```python
from build123d import *

# Parameters (mm, degrees)
SKETCH_R          = 20.32
SKETCH_R_2        = 2.225
PAD_DEPTH         = 36.83
FILLET_R          = 0.5
SKETCH001_R       = 1.05
PAD001_DEPTH      = 18.415
PAD001_DEPTH_BACK = 3.5


with BuildPart() as fillet_body:
    # Sketch → Pad (new body)
    with BuildSketch(Plane.XY.offset(0.1)):
        with Locations((14.35, 0)):
            Circle(SKETCH_R)
        with Locations((14.35, 0)):
            Circle(SKETCH_R_2, mode=Mode.SUBTRACT)
    extrude(amount=PAD_DEPTH)

    # Fillet
    fillet_edges = [fillet_body.edges().sort_by_distance(p)[0] for p in [
        (12.125, 0, 36.93),
        (-5.97, 0, 36.93),
        (-5.97, 0, 0.1),
    ]]
    fillet(fillet_edges, radius=FILLET_R)


with BuildPart() as obj1:
    # Sketch001 → Pad001 (new body, two sides)
    with BuildSketch(Plane.XY.offset(0.5)) as pad001_sk:
        Circle(SKETCH001_R)
        with Locations((28.7, 0)):
            Circle(SKETCH001_R)
    extrude(amount=PAD001_DEPTH)
    extrude(pad001_sk.sketch, amount=-PAD001_DEPTH_BACK)

    # obj1: union Fillet body
    add(fillet_body.part)


solid = obj1.part
```
Design review of the part built by this model. Coordinates are the model's own, in mm. A direction names the side the tool comes from. Round coordinates to 2 decimals unless told otherwise and drop trailing zeros. Write each loop counter-clockwise with the first axis right and the second up, starting at its lowest first coordinate (ties: lowest second). Pieces come first, ordered by that corner, then holes. Notation, with made-up numbers: (41.25, -3) -> (69.25, -3) arc R30 ccw to (69.25, 30) -> close; hole circle Ø10 at (43, 0). An arc over 180 degrees is marked (long way). Write item = value, one per line. Start each with the question number.
1) Tool access review of faces 1 (the face through (1, 0.32, -1.43)), 2 (the face through (16.47, 0.67, 18.01)): name each direction out of +Z, -Z, +X, -X, +Y, -Y from which nothing blocks a thin tool from reaching the whole face with its end or side.
2) Mouldability with a two-part tool opening along Z and no side actions: class faces 3 (the face through (18, 0, 0.1)), 4 (the face through (29.7, 0.32, -1.43)), 5 (the face through (14, -4, 36.93)) as +Z half, -Z half, draft (parallel to the pull), parting line (faces both ways), or undercut.
3) Clearance check with flat-ended pins moving along their axes: pin 1 (3 mm diameter, centred on x = 19, z = 2.5, fed in from +Y); pin 2 (10 mm diameter, centred on y = 10, z = 28.5, fed in from -X); pin 3 (1.5 mm diameter, centred on x = 24.5, z = 7.5, fed in from -Y). State where each tip first meets the part, or that it passes through.
4) Take a section at B-B, the plane x = 14.35. State the section outline as (y, z) points (3 decimals), plus the area to 3 significant figures.
5) Take a section at A-A, the plane y = 0. State the section outline as (x, z) points (3 decimals).
6) Wall thickness on probe 1 along Y at (x, z) = (14.35, 26) (3 decimals); probe 2 along Z at (x, y) = (9, 12.5); probe 3 along X at (y, z) = (-2, 28.5) (3 decimals): over which ranges is each line inside the solid? List them lowest first. Write a range as from..to.
7) Take a section at C-C, the plane z = 29.5. State the section outline as (x, y) points (3 decimals), plus the area to 3 significant figures.
Results list:
q1.face_1 = -Z
q1.face_2 = +Z, -Z
q2.face_3 = -Z half
q2.face_4 = draft
q2.face_5 = +Z half
q3.pin_1 = 20.07
q3.pin_2 = -5.35
q3.pin_3 = -18.02
q4.outline = (-20.32, 0.6) arc R0.5 ccw to (-19.82, 0.1) -> (-2.225, 0.1) -> (-2.225, 36.43) arc R0.5 ccw to (-2.725, 36.93) -> (-19.82, 36.93) arc R0.5 ccw to (-20.32, 36.43) -> close; (2.225, 0.1) -> (19.82, 0.1) arc R0.5 ccw to (20.32, 0.6) -> (20.32, 36.43) arc R0.5 ccw to (19.82, 36.93) -> (2.725, 36.93) arc R0.5 ccw to (2.225, 36.43) -> close
q4.area = 1,330 mm²
q5.outline = (-5.97, 0.6) arc R0.5 ccw to (-5.47, 0.1) -> (-1.05, 0.1) -> (-1.05, -3) -> (1.05, -3) -> (1.05, 0.1) -> (12.125, 0.1) -> (12.125, 36.43) arc R0.5 ccw to (11.625, 36.93) -> (-5.47, 36.93) arc R0.5 ccw to (-5.97, 36.43) -> close; (16.575, 0.1) -> (27.65, 0.1) -> (27.65, -3) -> (29.75, -3) -> (29.75, 0.1) -> (34.17, 0.1) arc R0.5 ccw to (34.67, 0.6) -> (34.67, 36.43) arc R0.5 ccw to (34.17, 36.93) -> (17.075, 36.93) arc R0.5 ccw to (16.575, 36.43) -> close
q6.probe_1 = -20.32..-2.225, 2.225..20.32
q6.probe_2 = 0.1..36.93
q6.probe_3 = -5.871..13.375, 15.325..34.571
q7.outline = circle Ø40.64 at (14.35, 0); hole circle Ø4.45 at (14.35, 0)
q7.area = 1,280 mm²
